Verification items for this drawing (mm, ordinates from the low corner). A direction names the side the tool comes from. Coordinates: 2 decimals unless noted, no trailing zeros. Write each loop counter-clockwise with the first axis right and the second up, starting at its lowest first coordinate (ties: lowest second). Pieces come first, ordered by that corner, then holes. Notation, with made-up numbers: (45, 85) -> (77, 85) arc R25 cw to (77, 102) -> close; hole circle Ø6 at (59.5, 7). An arc over 180 degrees is marked (long way). Put each result on its own line as item: value. Start each with the question number.
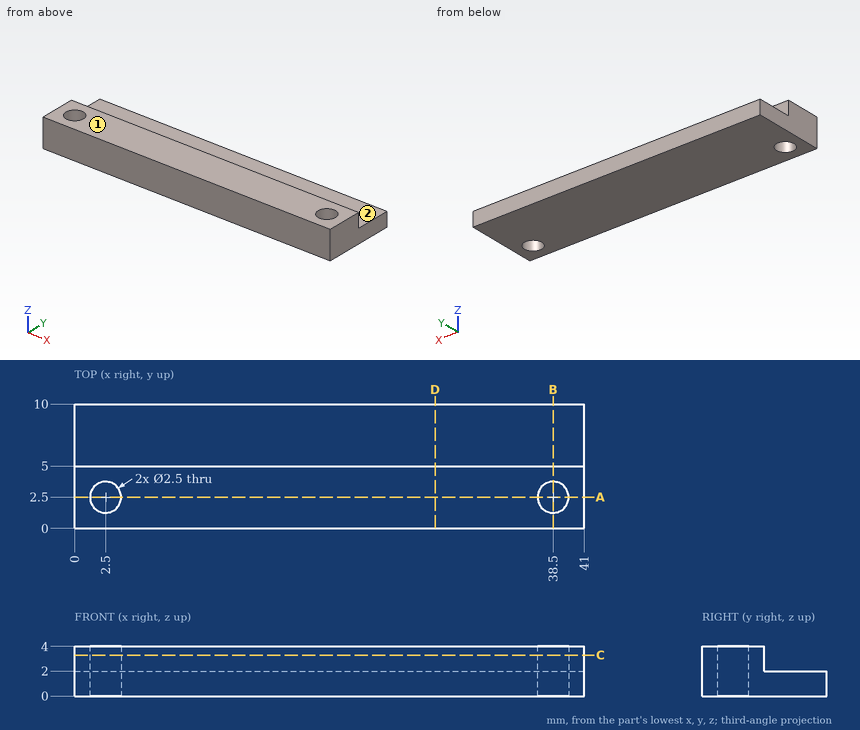
Item 1: Access from +Z, -Z, +X, -X, +Y, -Y to the whole of each face (thin tool, end or side, straight path). Record for the marked faces 1 and 2.
Item 2: Section check C-C, the plane z = 3.3. Enter the section's corners in (x, y), and give its area (3 significant figures).
Item 3: Scan lines: line 1 along Y through (x, z) = (2.5, 2.7); line 2 along X through (y, z) = (1.5, 2.6); line 3 along Y through (x, z) = (38.5, 0.9). Record each from-to range of solid material in increasing order. Write a range as [from, to].
Item 4: Section check D-D, the plane x = 29. Enter the section's corners in (y, z).
Item 5: Section check B-B, the plane x = 38.5. Enter the section's corners in (y, z), and give its area (3 significant figures).
Item 6: Section check A-A, the plane y = 2.5. Enter the section's corners in (x, z).
Item 7: Go/stop test with a flat-tipped pin: P1, Ø2, axis at x = 38.5, y = 2.5, coming from the -Z side. Record where the tip stops, or that it passes through.
From the geometry:
1. face 1: +Z, +X, -X, +Y, -Y
1. face 2: +Z, +X, -X, +Y
2. outline: (0, 0) -> (41, 0) -> (41, 5) -> (0, 5) -> close; hole circle Ø2.5 at (2.5, 2.5); hole circle Ø2.5 at (38.5, 2.5)
2. area: 195 mm²
3. line 1: [0, 1.25], [3.75, 5]
3. line 2: [0, 1.75], [3.25, 37.75], [39.25, 41]
3. line 3: [0, 1.25], [3.75, 10]
4. outline: (0, 0) -> (10, 0) -> (10, 2) -> (5, 2) -> (5, 4) -> (0, 4) -> close
5. outline: (0, 0) -> (1.25, 0) -> (1.25, 4) -> (0, 4) -> close; (3.75, 0) -> (10, 0) -> (10, 2) -> (5, 2) -> (5, 4) -> (3.75, 4) -> close
5. area: 20.0 mm²
6. outline: (0, 0) -> (1.25, 0) -> (1.25, 4) -> (0, 4) -> close; (3.75, 0) -> (37.25, 0) -> (37.25, 4) -> (3.75, 4) -> close; (39.75, 0) -> (41, 0) -> (41, 4) -> (39.75, 4) -> close
7. P1: through
